Design review of the part built by this model. Coordinates are the model's own, in mm. A direction names the side the tool comes from. Give positions to 0.01 mm unless a question says otherwise; leave off trailing zeros. Write each loop counter-clockwise with the first axis right and the second up, starting at its lowest first coordinate (ties: lowest second). Pieces come first, ordered by that corner, then holes. Notation, with made-up numbers: (73, -33.5) -> (102, -33.5) arc R27 ccw to (102, -6.5) -> close; hole circle Ø3 at (41.25, 19.5). An arc over 180 degrees is marked (long way). Return JSON: item names as keys, results as strings. Group by question number.
Autodesk Inventor part; units mm, degrees
ref_plane "YZ Plane" through (0, 0, 0) normal (1, 0, 0) x (0, 1, 0)
ref_plane "XZ Plane" through (0, 0, 0) normal (0, 1, 0) x (-1, 0, 0)
ref_plane "XY Plane" through (0, 0, 0) normal (0, 0, 1) x (1, 0, 0)
sketch "Sketch1" plane through (0, 0, 0) normal (0, 1, 0) x (-1, 0, 0)
  line L0 (0, 0) -> (100, 0)
  line L1 (100, 0) -> (100, -130)
  line L2 (100, -130) -> (0, -130)
  line L3 (0, -130) -> (0, 0)
  line L4 (61, -26.75) -> (19.5, -26.75) construction
  line L5 (19.5, -26.75) -> (19.5, -103.25) construction
  line L6 (19.5, -103.25) -> (61, -103.25) construction
  line L7 (61, -103.25) -> (61, -26.75) construction
  line L8 (61, -65) -> (19.5, -65) construction
  line L9 (70, 0) -> (30, 0)
  line L10 (30, 0) -> (30, -5)
  line L11 (30, -5) -> (70, -5)
  line L12 (70, -5) -> (70, 0)
  line L13 (70, -130) -> (30, -130)
  line L14 (30, -130) -> (30, -125)
  line L15 (30, -125) -> (70, -125)
  line L16 (70, -125) -> (70, -130)
  line L17 (61, -26.75) -> (51, -26.75)
  line L18 (51, -21.75) -> (66, -21.75)
  line L19 (66, -21.75) -> (66, -36.75)
  line L20 (66, -36.75) -> (61, -36.75)
  line L21 (61, -26.75) -> (61, -36.75)
  line L22 (51, -103.25) -> (51, -108.25)
  line L23 (51, -108.25) -> (66, -108.25)
  line L24 (66, -108.25) -> (66, -93.25)
  line L25 (66, -93.25) -> (61, -93.25)
  line L26 (61, -103.25) -> (61, -93.25)
  line L27 (61, -103.25) -> (51, -103.25)
  line L28 (82.3, -43.25) -> (61, -43.25) construction
  line L29 (61, -43.25) -> (61, -86.75) construction
  line L30 (61, -86.75) -> (82.3, -86.75) construction
  line L31 (82.3, -86.75) -> (82.3, -43.25) construction
  line L32 (82.3, -43.25) -> (82.3, -48.25)
  line L33 (87.05, -43.25) -> (82.3, -43.25)
  line L34 (82.3, -43.25) -> (61, -43.25)
  line L35 (61, -43.25) -> (61, -56.25)
  line L36 (61, -56.25) -> (82.3, -56.25)
  line L37 (82.3, -56.25) -> (82.3, -43.25)
  line L38 (82.3, -65) -> (61, -65) construction
  line L39 (82.3, -86.75) -> (61, -86.75)
  line L40 (61, -73.75) -> (82.3, -73.75)
  line L41 (82.3, -81.75) -> (82.3, -86.75)
  line L42 (61, -73.75) -> (61, -86.75)
  line L43 (51, -26.75) -> (51, -21.75)
  circle A0 centre (16, -65) radius 1.55
  line L44 (82.3, -73.75) -> (82.3, -81.75)
  line L45 (82.3, -72.5) -> (87.3, -72.5)
  line L46 (87.3, -72.5) -> (87.3, -57.5)
  line L47 (87.3, -57.5) -> (82.3, -57.5)
  line L48 (82.3, -57.5) -> (82.3, -72.5)
  line L49 (74.3, -86.75) -> (69.3, -86.75)
  line L50 (69.3, -86.75) -> (69.3, -91.75)
  line L51 (69.3, -91.75) -> (74.3, -91.75)
  line L52 (74.3, -91.75) -> (74.3, -86.75)
  line L53 (74.3, -43.25) -> (69.3, -43.25)
  line L54 (69.3, -43.25) -> (69.3, -38.25)
  line L55 (69.3, -38.25) -> (74.3, -38.25)
  line L56 (74.3, -38.25) -> (74.3, -43.25)
  point P0 (100, -65)
  point P1 (50, 0)
  point P2 (50, -5)
  point P3 (50, 0)
  point P4 (60, -115)
  point P5 (70, -115)
  point P6 (66, -29.25)
  point P7 (92.05, -81.75)
  point P8 (92.05, -48.25)
  point P9 (51, -105.75)
  point P10 (63.5, -93.25)
  point P11 (87.3, -65)
  point P12 (82.3, -84.25)
  point P13 (74.3, -89.25)
  point P14 (87.05, -43.25)
  point P15 (50, -130)
  point P16 (70, -2.5)
  point P17 (70, -127.5)
  dimension "d0" = 100
  dimension "d1" = 130
  dimension "d2" = 76.5
  dimension "d3" = 41.5
  dimension "d19" = 40
  dimension "d20" = 5
  dimension "d43" = 43.5
  dimension "d44" = 21.3
  dimension "d50" = 0
  dimension "d55" = 13
  dimension "d58" = 10
  dimension "d59" = 5
  dimension "d60" = 5
  dimension "d62" = 10
  dimension "d63" = 5
  dimension "d64" = 15
  dimension "d65" = 15
  dimension "d66" = 5
  dimension "d67" = 10
  dimension "d68" = 10
  dimension "d83" = 3.1
  dimension "d84" = 3.5
  dimension "d85" = 6.5
  dimension "d86" = 15
  dimension "d87" = 5
  dimension "d88" = 5
  dimension "d89" = 5
  dimension "d90" = 8
  dimension "d93" = 40
  dimension "d94" = 5
  dimension "d95" = 34
extrude "Extrusion2" add sketch "Sketch1" against normal blind 5 contours L0 L10 L11 L12 L1 L2 L16 L15 L14 L3 | L0 L12 L11 L10 | L14 L15 L16 L2 | L17 L43 L18 L19 L20 L21 | L27 L26 L25 L24 L23 L22 | L32 L37 L36 L35 L34 | L34 L54 L55 L56 | L39 L42 L40 L44 L41 | L52 L51 L50 L39 | A0 | L48 L47 L46 L45
extrude "Extrusion3" add sketch "Sketch1" along normal blind 35 contours L0 L12 L11 L10 | L14 L15 L16 L2
sketch "Sketch2" plane through (-100, -5, 0) normal (0, 0, 1) x (1, 0, 0)
  line L0 (30, 5) -> (70, 5)
  line L1 (40, 5) -> (60, 5)
  line L2 (60, 5) -> (60, 27)
  line L3 (60, 27) -> (40, 27)
  line L4 (40, 27) -> (40, 5)
  line L5 (41.25, 34) -> (58.75, 34) construction
  line L6 (30, 40) -> (70, 40)
  point P0 (100, 5)
  point P1 (50, 5)
  point P2 (50, 27)
  point P3 (50, 34)
  dimension "d31" = 20
  dimension "d34" = 7
  dimension "d42" = 17.5
  dimension "d92" = 13
extrude "Extrusion6" cut sketch "Sketch2" against normal through all
hole "Hole2" at (-58.75, 29, 0) at (-41.25, 29, 0) direction (0, 0, -1) diameter 3.1 end through all
extrude "Extrusion7" cut sketch "Sketch1" against normal through all contours L32 L37 L36 L35 L34 | L39 L42 L40 L44 L41 | A0
extrude "Extrusion9" add sketch "Sketch1" along normal blind 5 contours L17 L43 L18 L19 L20 L21 | L27 L26 L25 L24 L23 L22 | L34 L54 L55 L56 | L52 L51 L50 L39 | L48 L47 L46 L45
properties part number "Chasis 1"
Q1. Take a section at C-C, the plane z = -82. Give the boundary of the cut face in (x, y), plus the area to 4 significant figures.
Q2. Take a section at A-A, the plane x = -54.5. Give the boundary of the cut face in (y, z), plus the area to 3 significant figures.
Q3. Tool access review of faces 1 (the face through (-74.3, 2, -41)), 2 (the face through (-82.3, 2, -65)), 3 (the face through (-50, 22, -127)), 4 (the face through (-56, 2, -26.75)), 5 (the face through (-85, 2, -72.5)): name each direction out of +Z, -Z, +X, -X, +Y, -Y from which nothing blocks a thin tool from reaching the whole face with its end or side.
Q4. Mouldability with a two-part tool opening along Y and no side actions: class faces 6 (the face through (-60.287, 29.202, -127.535)), 7 (the face through (-72, 2, -91.75)), 8 (the face through (-50, 35, -2)) as +Y half, -Y half, draft (parallel to the pull), parting line (faces both ways), or undercut.
Q5. Insertion check: pin 1 (2.5 mm diameter, centred on x = -54.5, y = 3, fed in from +Z); pin 2 (1.5 mm diameter, centred on x = -71.5, y = 3, fed in from -Z); pin 3 (2.5 mm diameter, centred on x = -83.5, y = 3.5, fed in from -Z). Each pin has a flat end and moves straight along its axis. Give the tip position at first contact, or say it passes through.
Q6. Take a section at B-B, the plane y = 29. Give the boundary of the cut face in (x, z), plus the area to 3 significant figures.
Q7. For L1, parallel to X at y = 29, z = -126.25; L2, parallel to Y at x = -58.75, z = -127.9; L3, parallel to Z at x = -69, y = 9.5, list the stretches that pass through material, from the lowest coordinate up. Write a range as from..to.
Q8. Take a section at D-D, the plane y = 18. Give the boundary of the cut face in (x, z).
Final values:
{
 "1": {"outline": "(-100, -5) -> (-82.3, -5) -> (-82.3, 0) -> (-100, 0) -> close; (-61, -5) -> (0, -5) -> (0, 0) -> (-61, 0) -> close", "area": "393.5 mm²"},
 "2": {"outline": "(-5, -130) -> (0, -130) -> (0, -108.25) -> (5, -108.25) -> (5, -103.25) -> (0, -103.25) -> (0, -26.75) -> (5, -26.75) -> (5, -21.75) -> (0, -21.75) -> (0, 0) -> (-5, 0) -> close; (22, -130) -> (35, -130) -> (35, -125) -> (22, -125) -> close; (22, -5) -> (35, -5) -> (35, 0) -> (22, 0) -> close", "area": "830 mm²"},
 "3": {"face 1": "+Z, -Z, -X, +Y", "face 2": "+Z, -Z, +X, +Y", "face 3": "+Z, -Z", "face 4": "+X, +Y", "face 5": "-Z, +X, -X, +Y"},
 "4": {"face 6": "undercut", "face 7": "draft", "face 8": "+Y half"},
 "5": {"pin 1": "stops at z = -21.75", "pin 2": "stops at z = -91.75", "pin 3": "stops at z = -72.5"},
 "6": {"outline": "(-70, -130) -> (-60.3, -130) -> (-60.3, -125) -> (-70, -125) -> close; (-70, -5) -> (-60.3, -5) -> (-60.3, 0) -> (-70, 0) -> close; (-57.2, -130) -> (-42.8, -130) -> (-42.8, -125) -> (-57.2, -125) -> close; (-57.2, -5) -> (-42.8, -5) -> (-42.8, 0) -> (-57.2, 0) -> close; (-39.7, -130) -> (-30, -130) -> (-30, -125) -> (-39.7, -125) -> close; (-39.7, -5) -> (-30, -5) -> (-30, 0) -> (-39.7, 0) -> close", "area": "338 mm²"},
 "7": {"L1": "x = -70..-60.3, -57.2..-42.8, -39.7..-30", "L2": "y = -5..0, 22..27.45, 30.55..35", "L3": "z = -130..-125, -5..0"},
 "8": {"outline": "(-70, -130) -> (-60, -130) -> (-60, -125) -> (-70, -125) -> close; (-70, -5) -> (-60, -5) -> (-60, 0) -> (-70, 0) -> close; (-40, -130) -> (-30, -130) -> (-30, -125) -> (-40, -125) -> close; (-40, -5) -> (-30, -5) -> (-30, 0) -> (-40, 0) -> close"}
}
